Check sheet for the modelled part. Datum: model origin and axes. Units: mm. A direction names the side the tool comes from. Round coordinates to 2 decimals unless told otherwise and drop trailing zeros. Loops run counter-clockwise (first coordinate to the right, second up) from the corner with the lowest first, then second, coordinate; pieces in that order, holes last. Notation, with made-up numbers: M 77,-13 L 113,-13 A14 cw 113,0 Z; hole C -31,80.5 d7. An arc over 180 degrees is marked long. One line per question, with ' | ' between items. Start each with the question number.
(1) Thickness scan on probe 1 along X at (y, z) = (-19.5, 128); probe 2 along X at (y, z) = (-16, 102); probe 3 along Z at (x, y) = (-15, -27.5). Record the ranges inside material, lowest first. Write a range as [from, to].
(2) Section check A-A (x = -133.5). Record the boundary of the cut face in (y, z).
(3) Tool access check on faces 5 (the face through (-262.516, -15, 51)), 6 (the face through (-27.875, -13, 138)), 7 (the face through (-282.516, -13, 90)), 8 (the face through (-8, -15, 55.384)), 9 (the face through (-105, 2, 40.384)). Record the directions out of +Z, -Z, +X, -X, +Y, -Y that give a thin tool (end or side, any length) a straight path to the whole face; none if there is none.
(4) Go/stop test with flat-tipped pins: P1, Ø3, axis at x = -9.5, z = 51, coming from the -Y side; P2, Ø3, axis at x = -6, y = -15, coming from the -Z side. Record where each tip stops, or that it passes through.
(5) Section check B-B (y = -26). Count the separate pieces of the cut face and the enclosed holes in it, and give its area (3 significant figures).
(6) Section check D-D (z = 130). Record the boundary of the cut face in (x, y).
(7) Draft check along Y on faces 1 (the face through (-222, -20, 138)), 2 (the face through (-183, -30, 138)), 3 (the face through (-277.516, -15, 90)), 4 (the face through (-114.875, -13, 138)). Enter one of: +Y half, -Y half, draft (parallel to the pull), parting line (faces both ways), or undercut.
```python
from build123d import *

# Parameters (mm, degrees)
EXTRUDE_1_DEPTH     = 5
SKETCH_4_W          = 20
SKETCH_4_H          = 20
SKETCH_4_W_2        = 10
SKETCH_4_H_2        = 10
EXTRUDE_2_DEPTH     = 35
SKETCH_5_W          = 244.874710442
SKETCH_5_H          = 5
SKETCH_5_W_2        = 5
SKETCH_5_H_2        = 60
EXTRUDE_3_DEPTH     = 30
SKETCH_7_W          = 40
SKETCH_7_H          = 15
CUT_EXTRUDE_2_DEPTH = 5


with BuildPart() as part:
    # 草图2 → 凸台-拉伸1 (new body)
    with BuildSketch(Plane(origin=(0, 0, 0), x_dir=(1, 0, 0), z_dir=(0, 1, 0))):
        Polygon((-232.515561992, 29.211958859), (-232.515561992, -40.383972047), (-282.515561992, -40.383972047), (-282.515561992, -140.383972047), (2.125454159, -140.383972047), (2.125454159, -40.383972047), (-52.515561992, -40.383972047), (-52.515561992, 29.211958859), (-82.515561992, 29.211958859), (-82.515561992, -40.383972047), (-127.515561992, -40.383972047), (-127.515561992, 29.211958859), (-157.515561992, 29.211958859), (-157.515561992, -40.383972047), (-202.515561992, -40.383972047), (-202.515561992, 29.211958859), align=None)
    extrude(amount=EXTRUDE_1_DEPTH)

    # 草图4 → 凸台-拉伸2 (add)
    # profile 1 of 4: a face of its own
    with BuildSketch(Plane(origin=(0, 5, 0), x_dir=(1, 0, 0), z_dir=(0, 1, 0))):
        with Locations((-272.515561992, -50.383972047)):
            Rectangle(SKETCH_4_W, SKETCH_4_H)
        with Locations((-272.515561992, -50.383972047)):
            Rectangle(SKETCH_4_W_2, SKETCH_4_H_2, mode=Mode.SUBTRACT)
    # profile 2 of 4: a face of its own
    with BuildSketch(Plane(origin=(0, 5, 0), x_dir=(1, 0, 0), z_dir=(0, 1, 0))):
        with Locations((-272.515561992, -130.383972047)):
            Rectangle(SKETCH_4_W, SKETCH_4_H)
        with Locations((-272.515561992, -130.383972047)):
            Rectangle(SKETCH_4_W_2, SKETCH_4_H_2, mode=Mode.SUBTRACT)
    # profile 3 of 4: a face of its own
    with BuildSketch(Plane(origin=(0, 5, 0), x_dir=(1, 0, 0), z_dir=(0, 1, 0))):
        with Locations((-7.874545841, -50.383972047)):
            Rectangle(SKETCH_4_W, SKETCH_4_H)
        with Locations((-7.874545841, -50.383972047)):
            Rectangle(SKETCH_4_W_2, SKETCH_4_H_2, mode=Mode.SUBTRACT)
    # profile 4 of 4: a face of its own
    with BuildSketch(Plane(origin=(0, 5, 0), x_dir=(1, 0, 0), z_dir=(0, 1, 0))):
        with Locations((-7.874545841, -130.383972047)):
            Rectangle(SKETCH_4_W, SKETCH_4_H)
        with Locations((-7.874545841, -130.383972047)):
            Rectangle(SKETCH_4_W_2, SKETCH_4_H_2, mode=Mode.SUBTRACT)
    extrude(amount=-EXTRUDE_2_DEPTH)

    # 草图5 → 凸台-拉伸3 (add)
    with BuildSketch(Plane.XZ):
        with Locations((-140.311901062, 137.883972047)):
            Rectangle(SKETCH_5_W, SKETCH_5_H)
        with Locations((-280.015561992, 90.383972047)):
            Rectangle(SKETCH_5_W_2, SKETCH_5_H_2)
        with Locations((-0.374545841, 90.383972047)):
            Rectangle(SKETCH_5_W_2, SKETCH_5_H_2)
    extrude(amount=EXTRUDE_3_DEPTH)

    # 草图7 → 切除-拉伸2 (cut)
    with BuildSketch(Plane.XY.offset(140.383972047)):
        with Locations((-134.874545841, -12.5)):
            Rectangle(SKETCH_7_W, SKETCH_7_H)
        with Locations((-47.874545841, -12.5)):
            Rectangle(SKETCH_7_W, SKETCH_7_H)
        with Locations((-221.874545841, -12.5)):
            Rectangle(SKETCH_7_W, SKETCH_7_H)
    extrude(amount=-CUT_EXTRUDE_2_DEPTH, mode=Mode.SUBTRACT)


solid = part.part
```
The answers:
1) probe 1: [-282.52, -277.52], [-267.52, -262.52], [-17.87, -12.87], [-2.87, 2.13] | probe 2: [-282.52, -277.52], [-2.87, 2.13] | probe 3: [40.38, 60.38], [120.38, 140.38]
2) outline: M -30,135.38 L -20,135.38 L -20,140.38 L -30,140.38 Z; M -5,135.38 L 0,135.38 L 0,-29.21 L 5,-29.21 L 5,140.38 L -5,140.38 Z
3) face 5: -Z, -Y | face 6: +Z, -Z | face 7: +Z, -Z, -X, +Y, -Y | face 8: -Y | face 9: -Z, +Y, -Y
4) P1: y = 0 | P2: z = 40.38
5) separate pieces: 1 | enclosed holes: 4 | area: 3,020 mm²
6) outline: M -282.52,-30 L -277.52,-30 L -277.52,0 L -267.52,0 L -267.52,-30 L -262.52,-30 L -262.52,0 L -17.87,0 L -17.87,-30 L -12.87,-30 L -12.87,0 L -2.87,0 L -2.87,-30 L 2.13,-30 L 2.13,5 L -282.52,5 Z
7) face 1: undercut | face 2: -Y half | face 3: draft | face 4: undercut
